```python
from build123d import *

# Parameters (mm, degrees)
F0_W     = 57.15
F0_H     = 50.8
F1_DEPTH = 2.54
F2_R     = 5.08
F3_W     = 46.736
F3_H     = 40.386
F4_DEPTH = 5.08
F5_W     = 17.78
F5_H     = 5.08
F6_DEPTH = 2.54


with BuildPart() as f1:
    # F0 (on Top) → F1 (new body)
    with BuildSketch(Plane.XY):
        Rectangle(F0_W, F0_H)
    extrude(amount=F1_DEPTH)

    # F2
    f2_edges = [f1.edges().sort_by_distance(p)[0] for p in [
        (-28.575, 25.4, 1.27),
        (28.575, 25.4, 1.27),
        (28.575, -25.4, 1.27),
        (-28.575, -25.4, 1.27),
    ]]
    fillet(f2_edges, radius=F2_R)

    # F3 (on face) → F4 (join)
    with BuildSketch(Plane.XY.offset(2.54)):
        with BuildLine():
            Line((25.908, -20.32), (25.908, 20.32))
            ThreePointArc((25.908, 20.32), (25.201249, 22.026249), (23.495, 22.733))
            Line((23.495, 22.733), (-23.495, 22.733))
            ThreePointArc((-23.495, 22.733), (-25.201249, 22.026249), (-25.908, 20.32))
            Line((-25.908, 20.32), (-25.908, -20.32))
            ThreePointArc((-25.908, -20.32), (-25.201249, -22.026249), (-23.495, -22.733))
            Line((-23.495, -22.733), (23.495, -22.733))
            ThreePointArc((23.495, -22.733), (25.201249, -22.026249), (25.908, -20.32))
        make_face()
        Rectangle(F3_W, F3_H, mode=Mode.SUBTRACT)
    extrude(amount=F4_DEPTH)

    # F5 (on face) → F6 (cut, through all)
    with BuildSketch(Plane(origin=(-25.908, 0, 0), x_dir=(0, -1, 0), z_dir=(-1, 0, 0))):
        with Locations((0, 5.08)):
            Rectangle(F5_W, F5_H)
    extrude(amount=-F6_DEPTH, mode=Mode.SUBTRACT)


solid = f1.part
```
Source: CAD feature listing. Evaluate the final solid. Frame: model axes, mm. A direction names the side the tool comes from. Round coordinates to 2 decimals unless told otherwise and drop trailing zeros. Loops run counter-clockwise (first coordinate to the right, second up) from the corner with the lowest first, then second, coordinate; pieces in that order, holes last. Notation, with made-up numbers: M 31,-3 L 40,-3 A10 ccw 40,1 Z; hole C 88.5,27.5 d10. An arc over 180 degrees is marked long. Use a Markdown table: item, result. Add a question column.
1. Ray query, line 1 along X through (y, z) = (14, 4); line 2 along Y through (x, z) = (-2, 4.5); line 3 along Z through (x, y) = (5, -12.5). Return the intervals inside material, ascending. Write a range as [from, to].
2. Pull-direction query (X, two-part tool) for faces 1 (the cylindrical face through (27.1, 23.9, 1.3)), 2 (the flat face through (-25, -8.89, 5)), 3 (the flat face through (-23.368, 14, 5)); classes: +X half, -X half, draft (parallel to the pull), parting line (faces both ways), or undercut.
3. Contact query for flat-ended pins moving along their axis: pin 1 (2.5 mm diameter, centred on y = 3.5, z = 5.5, fed in from +X); pin 2 (1.5 mm diameter, centred on x = -2.5, z = 6, fed in from -Y); pin 3 (2 mm diameter, centred on x = -25, z = 4.5, fed in from +Y). Output: stop coordinate, or through.
4. Set-up query: faces 4 (the flat face through (-25.908, 15, 5)), 5 (the cylindrical face through (-25.22, -22.01, 5.04)), 6 (the cylindrical face through (25.22, 22.01, 5.04)). Return all of +Z, -Z, +X, -X, +Y, -Y with unobstructed straight access to the full face (end or side cutting, diameter ignored); none if empty.
5. Cut plane C-C, the plane x = -22. Output: boundary loops of the cut face in (y, z), and give its area (3 significant figures).
6. Cut plane B-B, the plane y = 14.5. Output: boundary loops of the cut face in (x, z) (3 decimals).
7. Cut plane D-D, the plane y = 8. Output: boundary loops of the cut face in (x, z) (3 decimals), and give its area (3 significant figures).
8. Cut plane A-A, the plane z = 5. Output: boundary loops of the cut face in (x, y) (3 decimals), and give its area (3 significant figures).
Solution:
| question | item | result |
|---|---|---|
| 1 | line 1 | x = [-25.91, -23.37], [23.37, 25.91] |
| 1 | line 2 | y = [-22.73, -20.19], [20.19, 22.73] |
| 1 | line 3 | z = [0, 2.54] |
| 2 | face 1 | +X half |
| 2 | face 2 | draft |
| 2 | face 3 | undercut |
| 3 | pin 1 | stops at x = 25.91 |
| 3 | pin 2 | stops at y = -22.73 |
| 3 | pin 3 | stops at y = 22.68 |
| 4 | face 4 | +Z, -X, +Y, -Y |
| 4 | face 5 | +Z, -X, -Y |
| 4 | face 6 | +Z, +X, +Y |
| 5 | outline | M -25.4,0 L 25.4,0 L 25.4,2.54 L 22.73,2.54 L 22.73,7.62 L 20.19,7.62 L 20.19,2.54 L -20.19,2.54 L -20.19,7.62 L -22.73,7.62 L -22.73,2.54 L -25.4,2.54 Z |
| 5 | area | 155 mm2 |
| 6 | outline | M -28.575,0 L 28.575,0 L 28.575,2.54 L 25.908,2.54 L 25.908,7.62 L 23.368,7.62 L 23.368,2.54 L -23.368,2.54 L -23.368,7.62 L -25.908,7.62 L -25.908,2.54 L -28.575,2.54 Z |
| 7 | outline | M -28.575,0 L 28.575,0 L 28.575,2.54 L 25.908,2.54 L 25.908,7.62 L 23.368,7.62 L 23.368,2.54 L -28.575,2.54 Z |
| 7 | area | 158 mm2 |
| 8 | outline | M -25.908,-20.32 A2.413 ccw -23.495,-22.733 L 23.495,-22.733 A2.413 ccw 25.908,-20.32 L 25.908,20.32 A2.413 ccw 23.495,22.733 L -23.495,22.733 A2.413 ccw -25.908,20.32 L -25.908,8.89 L -23.368,8.89 L -23.368,20.193 L 23.368,20.193 L 23.368,-20.193 L -23.368,-20.193 L -23.368,-8.89 L -25.908,-8.89 Z |
| 8 | area | 418 mm2 |
